Autodesk Inventor part; units mm, degrees
ref_plane "YZ Plane" through (0, 0, 0) normal (1, 0, 0) x (0, 1, 0)
ref_plane "XZ Plane" through (0, 0, 0) normal (0, 1, 0) x (-1, 0, 0)
ref_plane "XY Plane" through (0, 0, 0) normal (0, 0, 1) x (1, 0, 0)
sketch "Sketch1" plane through (0, 0, 0) normal (0, 1, 0) x (-1, 0, 0)
  circle A0 centre (8, -12.5) radius 1.1261
  line L0 (-4.5, -30.5) -> (20.5, -30.5)
  line L1 (20.5, -30.5) -> (20.5, 5.5)
  line L2 (20.5, 5.5) -> (-4.5, 5.5)
  line L3 (-4.5, 5.5) -> (-4.5, -30.5)
  line L4 (-4.5, -30.5) -> (20.5, 5.5) construction
  line L5 (20.5, -30.5) -> (-4.5, 5.5) construction
  dimension "d7" = 25
  dimension "d8" = 36
extrude "Extrusion1" add sketch "Sketch1" along normal blind 1
ref_plane "Work Plane1" through (16.9, 36.305, -11.9513) normal (0, 0.7071, 0.7071) x (-1, 0, 0)
sketch "Sketch2" plane through (16.9, 36.305, -11.9513) normal (0, 0.7071, 0.7071) x (-1, 0, 0)
  ellipse E0 centre (24.9, 24.5764) end of major axis (23.7739, 24.5764) minor radius 0.7963
  circle A0 centre (24.9, 24.9) radius 1.1798
  ellipse E1 centre (24.9, 25.2835) end of major axis (23.7739, 25.2835) minor radius 0.7963
  line L0 (12.4, 11.8485) -> (37.4, 11.8485)
  circle A1 centre (37.4, 11.8485) radius 1.2055
  circle A2 centre (12.4, 11.8485) radius 0.8893
  point P0 (16.9, 34.1223)
  dimension "d4" = 0.3236
extrude "Extrusion2" cut sketch "Sketch2" against normal through all contours E0 E1 A0 | E0 A0 E1 | E1 A0 E0 | E0 E1 | E0 A0 | E1 A0 E0 | A1 | A2 picked at (24.9476, 23.7672)
ref_plane "Work Plane2" through (-8, 0, -30.5) normal (-1, 0, 0) x (0, 0, 1)
ref_plane "Work Plane3" through (4, -7.358, 16.4985) normal (-0.7071, -0.5, 0.5) x (0.7071, -0.5, 0.5)
ref_plane "Work Plane4" through (4, -34.1432, -4.941) normal (0, -0.7071, 0.7071) x (1, 0, 0)
sketch "Sketch3" plane through (4, -34.1432, -4.941) normal (0, -0.7071, 0.7071) x (1, 0, 0)
  arc A0 (-13.1253, 18.7686) -> (-10.8747, 18.7686) centre (-12, 18.4144) ccw
  circle A1 centre (-12, 18.4144) radius 1.1798
  point P0 (-4, 27.6367)
extrude "Extrusion3" cut sketch "Sketch3" against normal through all
properties part number "00_Comar_Dichroic_16x25x0.2" material "Glas"
Here's how the part is built. I have some questions about the finished solid (model axes, mm). Round coordinates to 2 decimals unless told otherwise and drop trailing zeros. One line per question, with ' | ' between items.
1) For pin 1 Ø10 at (x, z) = (-7, -6.5) entering from -Y, with a flat end and sliding along its axis, tell me the tip position at first contact or that it passes through.
Working result:
pin 1: y = 0
2) I need wall thicknesses on line 1 along Z through (x, y) = (-7, 0.2); line 2 along X through (y, z) = (0.4, -11.5); line 3 along Z through (x, y) = (-7.25, 0.15). Which ranges of each line are inside material? Lowest first, please.
Working result:
line 1: -30.5 to -14.13, -11.96 to 5.5 | line 2: -20.5 to -8.86, -7.14 to 4.5 | line 3: -30.5 to -14.48, -11.6 to 5.5
3) If we mould it in two halves opening along X, with no side actions, what happens to faces 1 (the face through (-19.82, 0.48, -29.61)), 2 (the face through (-8.09, 0.17, -11.21)), 3 (the face through (-11, 0, -12))? For each: +X half, -X half, draft (parallel to the pull), parting line (faces both ways), or undercut.
Working result:
face 1: -X half | face 2: undercut | face 3: draft
